Here's how the part is built. I have some questions about the finished solid (model axes, mm). Face numbers are marked on the shaded views. A direction names the side the tool comes from. Round coordinates to 2 decimals unless told otherwise and drop trailing zeros. Loops run counter-clockwise (first coordinate to the right, second up) from the corner with the lowest first, then second, coordinate; pieces in that order, holes last. Notation, with made-up numbers: M 34,81 L 69,81 A11 ccw 69,93 Z; hole C 54,54.25 d7. An arc over 180 degrees is marked long. Answer as CSV lines item,"result".
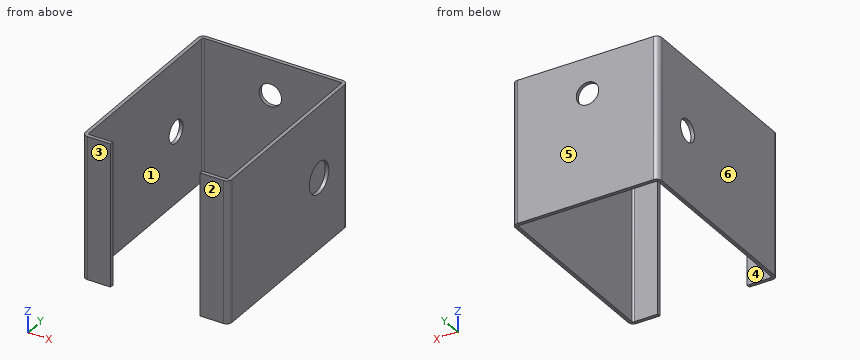
```python
from build123d import *

# Parameters (mm, degrees)
SKETCH2_W                    = 1.5875
SKETCH2_H                    = 82.55
BASE_FLANGE1_DEPTH           = 63.5
EDGE_FLANGE1_STRIP_W         = 7.8232
EDGE_FLANGE1_STRIP_H         = 1.5875
EDGE_FLANGE1_STRIP_CUT_DEPTH = 63.5
EDGE_FLANGE1_DEPTH           = 63.5
SKETCH10_R                   = 7
CUT_EXTRUDE1_DEPTH           = 105.73891424
EDGE_FLANGE2_STRIP_W         = 7.8232
EDGE_FLANGE2_STRIP_H         = 1.5875
EDGE_FLANGE2_STRIP_CUT_DEPTH = 63.5
EDGE_FLANGE2_DEPTH           = 63.5
EDGE_FLANGE3_STRIP_W         = 7.8232
EDGE_FLANGE3_STRIP_H         = 1.5875
EDGE_FLANGE3_STRIP_CUT_DEPTH = 63.5
EDGE_FLANGE3_DEPTH           = 63.5
EDGE_FLANGE4_STRIP_W         = 7.8232
EDGE_FLANGE4_STRIP_H         = 1.5875
EDGE_FLANGE4_STRIP_CUT_DEPTH = 63.5
EDGE_FLANGE4_DEPTH           = 63.5
SKETCH20_R                   = 5
CUT_EXTRUDE2_DEPTH           = 125.278268888
SKETCH21_R                   = 5
CUT_EXTRUDE3_DEPTH           = 9.652


# Sheet-metal steps are written as plain solids
with BuildPart() as part:
    # Sketch2 → Base-Flange1 (new body)
    with BuildSketch(Plane.XY):
        with Locations((0.79375, 41.275)):
            Rectangle(SKETCH2_W, SKETCH2_H)
    extrude(amount=BASE_FLANGE1_DEPTH)

    # Edge-Flange1 strip (across the edge) → Edge-Flange1 strip cut (cut)
    with BuildSketch(Plane(origin=(0, 0, 0), x_dir=(0, 1, 0), z_dir=(0, 0, 1))):
        with Locations((-3.175, -0.79375)):
            Rectangle(EDGE_FLANGE1_STRIP_W, EDGE_FLANGE1_STRIP_H)
    extrude(amount=EDGE_FLANGE1_STRIP_CUT_DEPTH, mode=Mode.SUBTRACT)

    # Edge-Flange1 section (across the edge) → Edge-Flange1 (add)
    with BuildSketch(Plane(origin=(0, 0, 0), x_dir=(0, 1, 0), z_dir=(0, 0, 1))):
        with BuildLine():
            Line((-1.5875, 0.7366), (-1.5875, 11.1125))
            Line((-1.5875, 11.1125), (0, 11.1125))
            Line((0, 11.1125), (0, 0.7366))
            ThreePointArc((0, 0.7366), (0.215745145, 0.215745145), (0.7366, 0))
            Line((0.7366, 0), (0.7366, -1.5875))
            ThreePointArc((0.7366, -1.5875), (-0.90678687, -0.90678687), (-1.5875, 0.7366))
        make_face()
    extrude(amount=EDGE_FLANGE1_DEPTH)

    # Sketch10 → Cut-Extrude1 (cut, through all)
    with BuildSketch(Plane.ZY):
        with Locations((31.75, 63.4125)):
            Circle(SKETCH10_R)
    extrude(amount=-CUT_EXTRUDE1_DEPTH, mode=Mode.SUBTRACT)

    # Edge-Flange2 strip (across the edge) → Edge-Flange2 strip cut (cut)
    with BuildSketch(Plane(origin=(0, 82.55, 63.5), x_dir=(0, -1, 0), z_dir=(0, 0, -1))):
        with Locations((-3.175, -0.79375)):
            Rectangle(EDGE_FLANGE2_STRIP_W, EDGE_FLANGE2_STRIP_H)
    extrude(amount=EDGE_FLANGE2_STRIP_CUT_DEPTH, mode=Mode.SUBTRACT)

    # Edge-Flange2 section (across the edge) → Edge-Flange2 (add)
    with BuildSketch(Plane(origin=(0, 82.55, 63.5), x_dir=(0, -1, 0), z_dir=(0, 0, -1))):
        with BuildLine():
            Line((-1.5875, 0.7366), (-1.5875, 62.162499944))
            Line((-1.5875, 62.162499944), (0, 62.162499944))
            Line((0, 62.162499944), (0, 0.7366))
            ThreePointArc((0, 0.7366), (0.215745145, 0.215745145), (0.7366, 0))
            Line((0.7366, 0), (0.7366, -1.5875))
            ThreePointArc((0.7366, -1.5875), (-0.90678687, -0.90678687), (-1.5875, 0.7366))
        make_face()
    extrude(amount=EDGE_FLANGE2_DEPTH)

    # Edge-Flange3 strip (across the edge) → Edge-Flange3 strip cut (cut)
    with BuildSketch(Plane(origin=(-62.162499944, 82.55, 63.5), x_dir=(1, 0, 0), z_dir=(0, 0, -1))):
        with Locations((-3.175, -0.79375)):
            Rectangle(EDGE_FLANGE3_STRIP_W, EDGE_FLANGE3_STRIP_H)
    extrude(amount=EDGE_FLANGE3_STRIP_CUT_DEPTH, mode=Mode.SUBTRACT)

    # Edge-Flange3 section (across the edge) → Edge-Flange3 (add)
    with BuildSketch(Plane(origin=(-62.162499944, 82.55, 63.5), x_dir=(1, 0, 0), z_dir=(0, 0, -1))):
        with BuildLine():
            Line((-1.5875, 0.7366), (-1.5875, 82.55))
            Line((-1.5875, 82.55), (0, 82.55))
            Line((0, 82.55), (0, 0.7366))
            ThreePointArc((0, 0.7366), (0.215745145, 0.215745145), (0.7366, 0))
            Line((0.7366, 0), (0.7366, -1.5875))
            ThreePointArc((0.7366, -1.5875), (-0.90678687, -0.90678687), (-1.5875, 0.7366))
        make_face()
    extrude(amount=EDGE_FLANGE3_DEPTH)

    # Edge-Flange4 strip (across the edge) → Edge-Flange4 strip cut (cut)
    with BuildSketch(Plane(origin=(-62.162499944, 0, 63.5), x_dir=(0, 1, 0), z_dir=(0, 0, -1))):
        with Locations((-3.175, -0.79375)):
            Rectangle(EDGE_FLANGE4_STRIP_W, EDGE_FLANGE4_STRIP_H)
    extrude(amount=EDGE_FLANGE4_STRIP_CUT_DEPTH, mode=Mode.SUBTRACT)

    # Edge-Flange4 section (across the edge) → Edge-Flange4 (add)
    with BuildSketch(Plane(origin=(-62.162499944, 0, 63.5), x_dir=(0, 1, 0), z_dir=(0, 0, -1))):
        with BuildLine():
            Line((-1.5875, 0.7366), (-1.5875, 11.1125))
            Line((-1.5875, 11.1125), (0, 11.1125))
            Line((0, 11.1125), (0, 0.7366))
            ThreePointArc((0, 0.7366), (0.215745145, 0.215745145), (0.7366, 0))
            Line((0.7366, 0), (0.7366, -1.5875))
            ThreePointArc((0.7366, -1.5875), (-0.90678687, -0.90678687), (-1.5875, 0.7366))
        make_face()
    extrude(amount=EDGE_FLANGE4_DEPTH)

    # Sketch20 → Cut-Extrude2 (cut, through all)
    with BuildSketch(Plane(origin=(0, 84.1375, 0), x_dir=(1, 0, 0), z_dir=(0, 1, 0))):
        with Locations(Location((-32, -47.64999995, 0), (0, 0, 180))):
            Circle(SKETCH20_R)
    extrude(amount=-CUT_EXTRUDE2_DEPTH, mode=Mode.SUBTRACT)

    # Sketch21 → Cut-Extrude3 (cut)
    with BuildSketch(Plane(origin=(-62.162499944, 0, 0), x_dir=(0, 0, -1), z_dir=(1, 0, 0))):
        with Locations(Location((-31.75, 63.4125, 0), (0, 0, 90))):
            Circle(SKETCH21_R)
    extrude(amount=-CUT_EXTRUDE3_DEPTH, mode=Mode.SUBTRACT)


solid = part.part
```
1. We'd pull the mould along Y, two halves only. Please class the marked faces 3, 4, 5 and 6: pulls with the +Y half, pulls with the -Y half, needs draft (parallel to the pull), parting line crosses it, or undercut.
Evaluation:
face 3,"pulls with the -Y half"
face 4,"undercut"
face 5,"pulls with the +Y half"
face 6,"needs draft"
2. For P1, Ø1.3, axis at y = -0.5, z = 27, coming from the -X side; P2, Ø16, axis at y = 63.41, z = 31.75, coming from the +X side; P3, Ø0.8, axis at y = -0.5, z = 40.5, coming from the +X side, each with a flat end and sliding along its axis, tell me the tip position at first contact or that it passes through.
Evaluation:
P1,"stops at x = -63.67"
P2,"stops at x = 1.59"
P3,"stops at x = 1.43"
3. I want a section at C-C, the plane z = 47.65. Please give me the cut outline in (x, y), and give its area (3 significant figures).
Evaluation:
outline,"M -63.75,0.74 A2.32 ccw -61.43,-1.59 L -51.05,-1.59 L -51.05,0 L -61.43,0 A0.74 cw -62.16,0.74 L -62.16,81.81 A0.74 cw -61.43,82.55 L -37,82.55 L -37,84.14 L -61.43,84.14 A2.32 ccw -63.75,81.81 Z; M -27,82.55 L -0.74,82.55 A0.74 cw 0,81.81 L 0,0.74 A0.74 cw -0.74,0 L -11.11,0 L -11.11,-1.59 L -0.74,-1.59 A2.32 ccw 1.59,0.74 L 1.59,81.81 A2.32 ccw -0.74,84.14 L -27,84.14 Z"
area,"386 mm²"
4. If I drill on line 1 (X direction, y = 63.5, z = 20); line 2 (Z direction, x = -32, y = 83); line 3 (Y direction, x = -12.5, z = 34), over which ranges is the centre line in solid material (lowest first)? Write a range as [from, to].
Evaluation:
line 1,"x = [-63.75, -62.16], [0, 1.59]"
line 2,"z = [0, 42.65], [52.65, 63.5]"
line 3,"y = [82.55, 84.14]"
5. I want a section at A-A, the plane x = -32. Please give me the cut outline in (y, z).
Evaluation:
outline,"M 82.55,0 L 84.14,0 L 84.14,42.65 L 82.55,42.65 Z; M 82.55,52.65 L 84.14,52.65 L 84.14,63.5 L 82.55,63.5 Z"
6. I want a section at B-B, the plane y = 74. Please give me the cut outline in (x, z).
Evaluation:
outline,"M -63.75,0 L -62.16,0 L -62.16,63.5 L -63.75,63.5 Z; M 0,0 L 1.59,0 L 1.59,63.5 L 0,63.5 Z"
7. Which directions (+Z, -Z, +X, -X, +Y, -Y) give clear straight access to the entire face, cutting with the end or side of a thin tool? Please do the marked faces 1 and 2.
Evaluation:
face 1,"+Z, -Z"
face 2,"+Z, -Z, +X, -X, -Y"
8. I want a section at D-D, the plane z = 31.75. Please give me the cut outline in (x, y), and give its area (3 significant figures).
Evaluation:
outline,"M -63.75,0.74 A2.32 ccw -61.43,-1.59 L -51.05,-1.59 L -51.05,0 L -61.43,0 A0.74 cw -62.16,0.74 L -62.16,58.41 L -63.75,58.41 Z; M -63.75,68.41 L -62.16,68.41 L -62.16,81.81 A0.74 cw -61.43,82.55 L -0.74,82.55 A0.74 cw 0,81.81 L 0,70.41 L 1.59,70.41 L 1.59,81.81 A2.32 ccw -0.74,84.14 L -61.43,84.14 A2.32 ccw -63.75,81.81 Z; M -11.11,-1.59 L -0.74,-1.59 A2.32 ccw 1.59,0.74 L 1.59,56.41 L 0,56.41 L 0,0.74 A0.74 cw -0.74,0 L -11.11,0 Z"
area,"364 mm²"
